Verification items for the finished model (mm, model axes). A direction names the side the tool comes from. Coordinates: 2 decimals unless noted, no trailing zeros. Order: outer loops, then holes, each group sorted by start corner. A loop starts at its lowest first (then second) coordinate and runs counter-clockwise, first axis right, second up. Notation, with made-up numbers: M 3,28 L 42,28 A14 ccw 42,49 Z; hole C -30.75,-37.5 d4. An arc over 180 degrees is marked long. Answer as a JSON object with one key per item and string values. Group by question number.
(1) Access from +Z, -Z, +X, -X, +Y, -Y to the whole of each face (thin tool, end or side, straight path). Record for faces 5 (the face through (26, -3, 4)), 6 (the face through (-2, -25, 4)).
(2) Cross-section at B-B (z = 5.5). Count the separate pieces of the cut face and the enclosed holes in it, plus the area to 3 significant figures.
(3) Cross-section at A-A (y = -7.5). Enter the section's corners in (x, z).
(4) Gauge pin test, flat ends, axial feed: pin 1 Ø1 at (y, z) = (-21.5, 2.5) entering from +X; pin 2 Ø4 at (x, y) = (22.5, 0) entering from +Z; pin 3 Ø4 at (x, y) = (30, 0) entering from -Z. Record the tip position at first contact, or that the pin passes through.
(5) Mould release check, pull along X, two halves, no side actions. Record for faces 1 (the face through (-3, -11, 4)), 2 (the face through (47.248, 2.287, 3.944)), 3 (the face through (28.4, 0.07, 3.96)), 4 (the face through (36.32, 1.08, 3.96)): released by +X, released by -X, zero draft, split by the parting line, or undercut.
(6) Material ranges on line 1 (Y direction, x = 0, z = 1); line 2 (Y direction, x = 45, z = 2.9); line 3 (X direction, y = -20.75, z = 4.75), recorded low to high.
from build123d import *

# Parameters (mm, degrees)
SKETCH1_R           = 1.6
BOSS_EXTRUDE1_DEPTH = 8
CHAMFER1_SIZE       = 1
SKETCH2_R           = 1.6
BOSS_EXTRUDE3_DEPTH = 8
FILLET1_R           = 2
CHAMFER3_SIZE       = 1
CHAMFER5_SIZE       = 1


with BuildPart() as part:
    # Sketch1 → Boss-Extrude1 (new body)
    with BuildSketch(Plane.XY):
        with BuildLine():
            Line((-0.5, 3), (45.5, 3))
            ThreePointArc((45.5, 3), (47.267766953, 2.267766953), (48, 0.5))
            Line((48, 0.5), (48, -0.5))
            ThreePointArc((48, -0.5), (47.267766953, -2.267766953), (45.5, -3))
            Line((45.5, -3), (-0.5, -3))
            ThreePointArc((-0.5, -3), (-2.267766953, -2.267766953), (-3, -0.5))
            Line((-3, -0.5), (-3, 0.5))
            ThreePointArc((-3, 0.5), (-2.267766953, 2.267766953), (-0.5, 3))
        make_face()
        Circle(SKETCH1_R, mode=Mode.SUBTRACT)
        with Locations((7.5, 0)):
            Circle(SKETCH1_R, mode=Mode.SUBTRACT)
        with Locations((15, 0)):
            Circle(SKETCH1_R, mode=Mode.SUBTRACT)
        with Locations((22.5, 0)):
            Circle(SKETCH1_R, mode=Mode.SUBTRACT)
        with Locations((30, 0)):
            Circle(SKETCH1_R, mode=Mode.SUBTRACT)
        with Locations((37.5, 0)):
            Circle(SKETCH1_R, mode=Mode.SUBTRACT)
        with Locations((45, 0)):
            Circle(SKETCH1_R, mode=Mode.SUBTRACT)
    extrude(amount=BOSS_EXTRUDE1_DEPTH)

    # Chamfer1
    chamfer1_edges = [part.edges().sort_by_distance(p)[0] for p in [
        (-1.6, 0, 0),
        (-1.6, 0, 8),
        (5.9, 0, 0),
        (5.9, 0, 8),
        (13.4, 0, 0),
        (13.4, 0, 8),
        (20.9, 0, 0),
        (20.9, 0, 8),
        (28.4, 0, 0),
        (28.4, 0, 8),
    ]]
    chamfer(chamfer1_edges, length=CHAMFER1_SIZE)

    # Sketch2 → Boss-Extrude3 (add)
    with BuildSketch(Plane.XY.offset(8)):
        with BuildLine():
            ThreePointArc((-0.5, -3), (-2.267766953, -2.267766953), (-3, -0.5))
            Line((-3, -0.5), (-3, -23))
            ThreePointArc((-3, -23), (-2.267766953, -24.767766953), (-0.5, -25.5))
            Line((-0.5, -25.5), (0.5, -25.5))
            ThreePointArc((0.5, -25.5), (2.267766953, -24.767766953), (3, -23))
            Line((3, -23), (3, -3))
            Line((3, -3), (-0.5, -3))
        make_face()
        with Locations((0, -22.5)):
            Circle(SKETCH2_R, mode=Mode.SUBTRACT)
        with Locations((0, -15)):
            Circle(SKETCH2_R, mode=Mode.SUBTRACT)
        with Locations((0, -7.5)):
            Circle(SKETCH2_R, mode=Mode.SUBTRACT)
    extrude(amount=-BOSS_EXTRUDE3_DEPTH)

    # Fillet1
    fillet1_edges = [part.edges().sort_by_distance(p)[0] for p in [
        (3, -3, 4),
    ]]
    fillet(fillet1_edges, radius=FILLET1_R)

    # Chamfer3
    chamfer3_edges = [part.edges().sort_by_distance(p)[0] for p in [
        (35.9, 0, 0),
        (35.9, 0, 8),
        (43.4, 0, 0),
        (43.4, 0, 8),
    ]]
    chamfer(chamfer3_edges, length=CHAMFER3_SIZE)

    # Chamfer5
    chamfer5_edges = [part.edges().sort_by_distance(p)[0] for p in [
        (-1.6, -7.5, 8),
        (-1.6, -15, 8),
        (-1.6, -22.5, 8),
        (-1.6, -22.5, 0),
        (-1.6, -15, 0),
        (-1.6, -7.5, 0),
    ]]
    chamfer(chamfer5_edges, length=CHAMFER5_SIZE)


solid = part.part
Taken from the geometry:
{
 "1": {"face 5": "+Z, -Z, +X, -Y", "face 6": "+Z, -Z, -X, -Y"},
 "2": {"separate pieces": "1", "enclosed holes": "10", "area": "355 mm²"},
 "3": {"outline": "M -3,0 L -2.6,0 L -1.6,1 L -1.6,7 L -2.6,8 L -3,8 Z; M 1.6,1 L 2.6,0 L 3,0 L 3,8 L 2.6,8 L 1.6,7 Z"},
 "4": {"pin 1": "stops at x = 3", "pin 2": "stops at z = 7.4", "pin 3": "stops at z = 0.6"},
 "5": {"face 1": "released by -X", "face 2": "released by +X", "face 3": "undercut", "face 4": "undercut"},
 "6": {"line 1": "y = -25.5 to -24.1, -20.9 to -16.6, -13.4 to -9.1, -5.9 to -1.6, 1.6 to 3", "line 2": "y = -3 to -1.6, 1.6 to 3", "line 3": "x = -3 to 3"}
}
